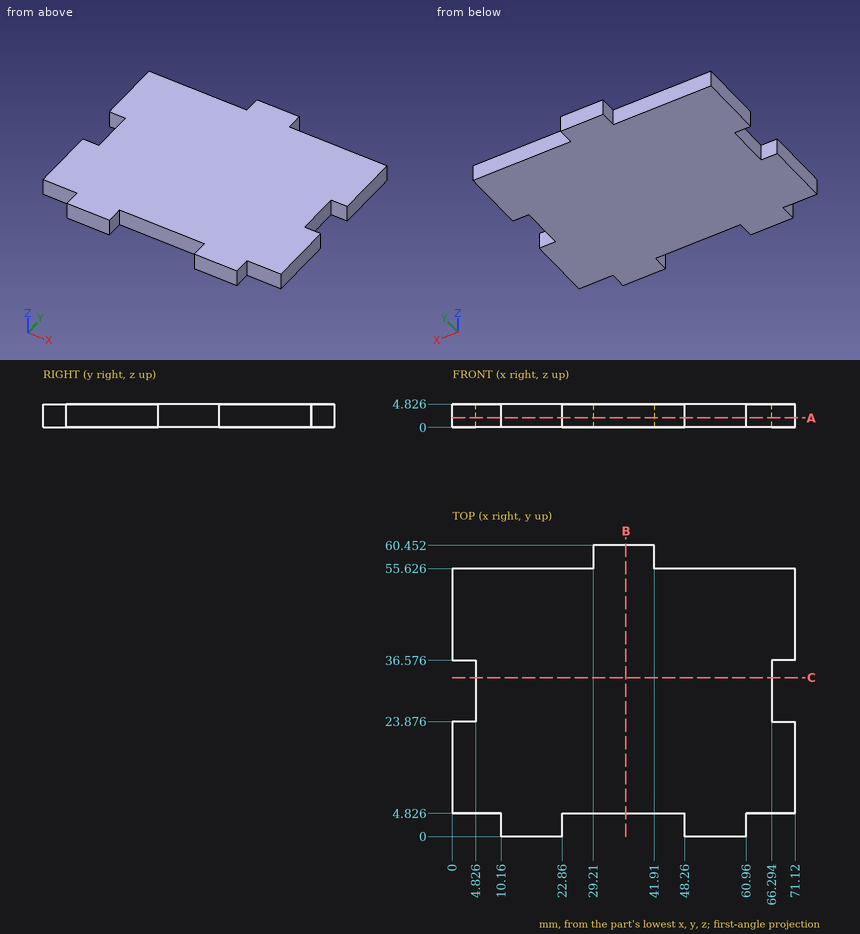
Verification items for this drawing (mm, ordinates from the low corner). Coordinates: 2 decimals unless noted, no trailing zeros. Write each loop counter-clockwise with the first axis right and the second up, starting at its lowest first coordinate (ties: lowest second). Pieces come first, ordered by that corner, then holes. Notation, with made-up numbers: M 69.5,-28.5 L 127.5,-28.5 A20 cw 127.5,-13.5 Z; hole C 32,4.25 d3. An arc over 180 degrees is marked long. Use one line per item in the form item = value. Start each with the question number.
1) Section check A-A on z = 1.95. Enter the section's corners in (x, y), and give its area (3 significant figures).
2) Section check B-B on x = 36. Enter the section's corners in (y, z), and give its area (3 significant figures).
3) Section check C-C on y = 33. Enter the section's corners in (x, z).
4) Thickness scan on probe 1 along Y at (x, z) = (17.5, 2.05); probe 2 along X at (y, z) = (29, 3.2); probe 3 along Y at (x, z) = (28, 3.55). Record the ranges inside material, lowest first. Write a range as from..to.
5) Go/stop test with flat-tipped pins: pin 1 Ø1.4 at (y, z) = (58.5, 1.5) entering from +X; pin 2 Ø1.4 at (x, z) = (67.5, 2.5) entering from -Y; pin 3 Ø1 at (y, z) = (33.5, 4) entering from -X. Record where each tip stops, or that it passes through.
Responses:
q1.outline = M 0,4.83 L 10.16,4.83 L 10.16,0 L 22.86,0 L 22.86,4.83 L 48.26,4.83 L 48.26,0 L 60.96,0 L 60.96,4.83 L 71.12,4.83 L 71.12,23.88 L 66.29,23.88 L 66.29,36.58 L 71.12,36.58 L 71.12,55.63 L 41.91,55.63 L 41.91,60.45 L 29.21,60.45 L 29.21,55.63 L 0,55.63 L 0,36.58 L 4.83,36.58 L 4.83,23.88 L 0,23.88 Z
q1.area = 3,670 mm2
q2.outline = M 4.83,0 L 60.45,0 L 60.45,4.83 L 4.83,4.83 Z
q2.area = 268 mm2
q3.outline = M 4.83,0 L 66.29,0 L 66.29,4.83 L 4.83,4.83 Z
q4.probe_1 = 0..55.63
q4.probe_2 = 4.83..66.29
q4.probe_3 = 4.83..55.63
q5.pin_1 = 41.91
q5.pin_2 = 4.83
q5.pin_3 = 4.83
